from build123d import *

# Parameters (mm, degrees)
F0_R     = 7.5
F0_R_2   = 1.5
F0_R_3   = 1
F1_DEPTH = 10
F2_DEPTH = 6
F3_R     = 15
F3_R_2   = 7.5
F4_DEPTH = 10
F5_R     = 4.99999


# Not quite as in the source:
# - a fillet or chamfer is up to 0.001 mm smaller than in the source, because OpenCascade refuses the exact size


with BuildPart() as f1:
    # F0 (on Top) → F1 (new body)
    with BuildSketch(Plane.XY):
        Circle(F0_R)
        Circle(F0_R_2, mode=Mode.SUBTRACT)
        Circle(F0_R_2)
        Circle(F0_R_3, mode=Mode.SUBTRACT)
        Circle(F0_R_3)
    extrude(amount=F1_DEPTH)

    # F0 (on Top) → F2 (join)
    with BuildSketch(Plane.XY):
        Circle(F0_R_2)
        Circle(F0_R_3, mode=Mode.SUBTRACT)
        Circle(F0_R_3)
    extrude(amount=-F2_DEPTH)

    # F3 (on face) → F4 (join)
    with BuildSketch(Plane.XY.offset(10)):
        Circle(F3_R)
        Circle(F3_R_2, mode=Mode.SUBTRACT)
        Circle(F3_R_2)
    extrude(amount=F4_DEPTH)

    # F5 (radius 5 in the source; OpenCascade refuses exactly that, so slightly less here)
    f5_edges = [f1.edges().sort_by_distance(p)[0] for p in [
        (15, 0, 15),
        (-15, 0, 10),
        (-15, 0, 20),
    ]]
    fillet(f5_edges, radius=F5_R)


solid = f1.part
Geometry: final body of the model. Coordinates: model frame, mm. A direction names the side the tool comes from. Coordinates: 2 decimals unless noted, no trailing zeros. Write each loop counter-clockwise with the first axis right and the second up, starting at its lowest first coordinate (ties: lowest second). Pieces come first, ordered by that corner, then holes. Notation, with made-up numbers: (-31, 70) - (-11, 70) arc R10 cw to (-11, 87) - close; hole circle Ø5 at (23.25, 60). An arc over 180 degrees is marked (long way). Return JSON: item names as keys, results as strings.
Item 1: Pin query (flat end, axial travel): pin 1 Ø6 at (x, y) = (2.5, -5) entering from -Z; pin 2 Ø1.5 at (x, y) = (8.5, 6) entering from -Z; pin 3 Ø5 at (y, z) = (8.5, 5) entering from +X. Return the tip coordinate at first contact, or that it passes through.
Completed:
{"pin 1": "stops at z = 0", "pin 2": "stops at z = 10", "pin 3": "stops at x = 4.5"}
Item 2: Section query C-C (z = 7.75). Output: boundary loops of the cut face in (x, y), and give its area (3 significant figures).
Completed:
{"outline": "circle Ø15 at (0, 0)", "area": "177 mm2"}
Item 3: Reachability of faces 1 (the face through (0, 0, 20)), 2 (the face through (-1.5, 0.07, -2.96)) from +Z, -Z, +X, -X, +Y, -Y: full face, straight path, thin tool, end or side. Return the list, or none.
Completed:
{"face 1": "+Z, +X, -X, +Y, -Y", "face 2": "-Z"}
Item 4: Section query D-D (z = -1.5). Output: boundary loops of the cut face in (x, y).
Completed:
{"outline": "circle Ø3 at (0, 0)"}
Item 5: Line query: L1, parallel to Z at x = -1, y = -10; L2, parallel to Z at x = 1, y = -4.5; L3, parallel to Y at x = -4, z = 9.25. Output: solid intervals per line, ascending.
Completed:
{"L1": "z = 10 to 20", "L2": "z = 0 to 20", "L3": "y = -6.34 to 6.34"}
